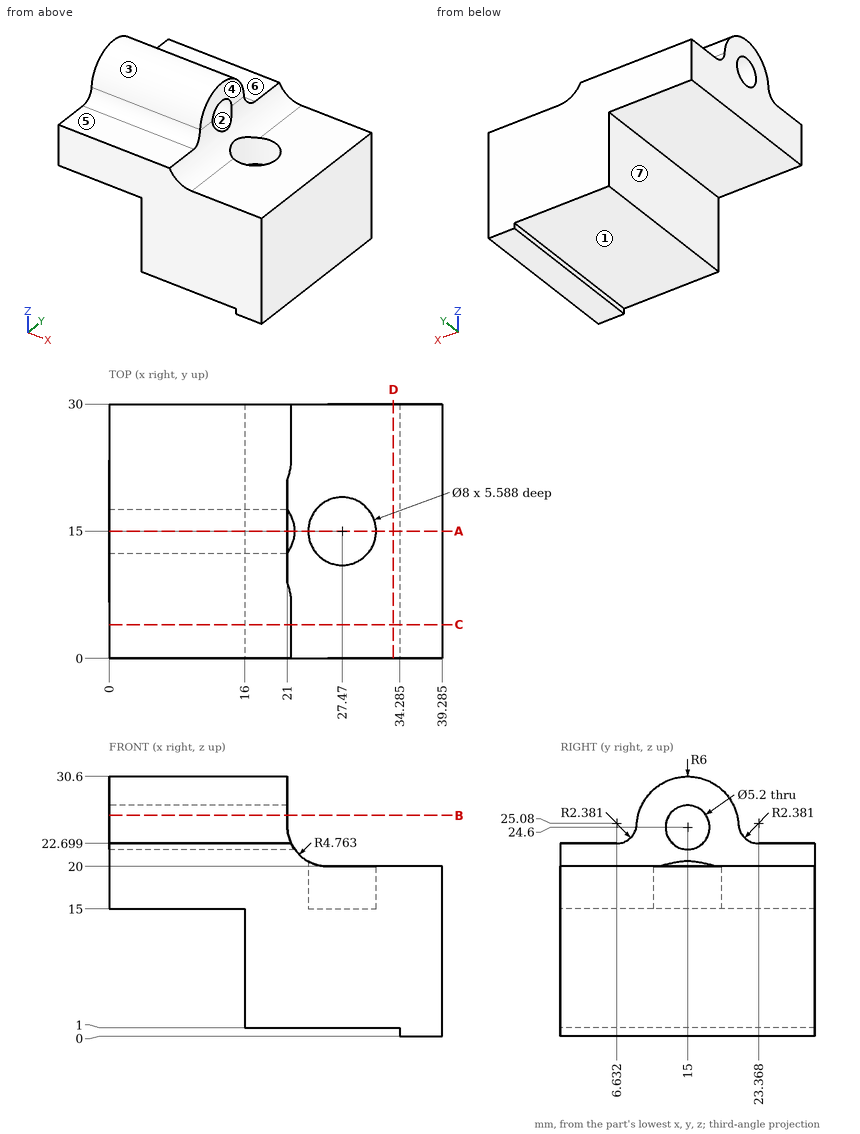
Print and shaded views of the part. All mm, measured from the part's lowest x, y and z. A direction names the side the tool comes from. Coordinates: 2 decimals unless noted, no trailing zeros. Order: outer loops, then holes, each group sorted by start corner. A loop starts at its lowest first (then second) coordinate and runs counter-clockwise, first axis right, second up.
Item 1: Saw through at D-D on x = 33.5. List the corners of the cut face in (y, z), then the cut area to 3 significant figures.
Filled in:
outline: (0, 1) - (30, 1) - (30, 20) - (0, 20) - close
area: 570 mm2
Item 2: Drop flat-ended pins along their axis: pin 1 Ø4 at (x, y) = (8, 22) entering from -Z; pin 2 Ø2 at (x, y) = (5.5, 26.5) entering from +Z; pin 3 Ø7 at (y, z) = (10.5, 10) entering from -X. Give the stop position or say it passes through.
Filled in:
pin 1: stops at z = 15
pin 2: stops at z = 22.7
pin 3: stops at x = 16
Item 3: Saw through at B-B on z = 26. List the corners of the cut face in (x, y) (1 decimal).
Filled in:
outline: (0, 9.2) - (21, 9.2) - (21, 12.8) - (0, 12.8) - close; (0, 17.2) - (21, 17.2) - (21, 20.8) - (0, 20.8) - close
Item 4: Mould opens along Z. For the marked faces 1, 2 and 3 say: released by +Z, released by -Z, zero draft, split by the parting line, or undercut.
Filled in:
face 1: released by -Z
face 2: undercut
face 3: released by +Z
Item 5: Tool access for the marked faces 4, 5, 6 and 7: list every direction of +Z, -Z, +X, -X, +Y, -Y with a clear straight run to the whole face (end or side of a thin tool).
Filled in:
face 4: +Z, +X, +Y, -Y
face 5: +Z, +X, -X, -Y
face 6: +Z, +X, -X, +Y
face 7: -Z, -X, +Y, -Y
Item 6: Drill centre lines: L1, parallel to Y at x = 5.5, z = 24.6 (1 decimal); L2, parallel to Z at x = 32.5, y = 27; L3, parallel to Y at x = 11, z = 24 (1 decimal). Where is each one in solid material? Low to high.
Filled in:
L1: y = 9 to 12.4, 17.6 to 21
L2: z = 1 to 20
L3: y = 8.8 to 12.5, 17.5 to 21.2
Item 7: Saw through at A-A on y = 15. List the corners of the cut face in (x, z) (1 decimal).
Filled in:
outline: (0, 15) - (16, 15) - (16, 1) - (34.3, 1) - (34.3, 0) - (39.3, 0) - (39.3, 20) - (31.5, 20) - (31.5, 15) - (23.5, 15) - (23.5, 20.6) arc R4.8 cw to (21.9, 22) - (0, 22) - close; (0, 27.2) - (21, 27.2) - (21, 30.6) - (0, 30.6) - close
Item 8: Saw through at C-C on y = 4. List the corners of the cut face in (x, z) (1 decimal).
Filled in:
outline: (0, 15) - (16, 15) - (16, 1) - (34.3, 1) - (34.3, 0) - (39.3, 0) - (39.3, 20) - (25.8, 20) arc R4.8 cw to (21.5, 22.7) - (0, 22.7) - close
